```python
from build123d import *

# Parameters (mm, degrees)
F0_W     = 303
F0_H     = 174
F0_R     = 9
F0_R_2   = 7.8
F0_W_2   = 43
F0_H_2   = 80
F0_W_3   = 16.5
F0_H_3   = 7.6
F1_DEPTH = 1


with BuildPart() as f1:
    # F0 (on Top) → F1 (new body)
    with BuildSketch(Plane.XY):
        Rectangle(F0_W, F0_H)
        with Locations((121.5, -57)):
            Circle(F0_R, mode=Mode.SUBTRACT)
        with Locations((21.5, -30)):
            Circle(F0_R_2, mode=Mode.SUBTRACT)
        with Locations((51.5, -30)):
            Circle(F0_R_2, mode=Mode.SUBTRACT)
        with Locations((-110, 27)):
            Rectangle(F0_W_2, F0_H_2, mode=Mode.SUBTRACT)
        with Locations((-37, 27)):
            Rectangle(F0_W_2, F0_H_2, mode=Mode.SUBTRACT)
        with Locations((21.5, 0)):
            Circle(F0_R_2, mode=Mode.SUBTRACT)
        with Locations((51.5, 0)):
            Circle(F0_R_2, mode=Mode.SUBTRACT)
        with Locations((21.5, 30)):
            Circle(F0_R_2, mode=Mode.SUBTRACT)
        with Locations((51.5, 30)):
            Circle(F0_R_2, mode=Mode.SUBTRACT)
        with Locations((89.75, 0)):
            Rectangle(F0_W_3, F0_H_3, mode=Mode.SUBTRACT)
        with Locations((89.75, 20)):
            Rectangle(F0_W_3, F0_H_3, mode=Mode.SUBTRACT)
        with Locations((89.75, 40)):
            Rectangle(F0_W_3, F0_H_3, mode=Mode.SUBTRACT)
        with Locations((21.5, 60)):
            Circle(F0_R_2, mode=Mode.SUBTRACT)
        with Locations((51.5, 60)):
            Circle(F0_R_2, mode=Mode.SUBTRACT)
        with Locations((89.75, 60)):
            Rectangle(F0_W_3, F0_H_3, mode=Mode.SUBTRACT)
    extrude(amount=F1_DEPTH)


solid = f1.part
```
Geometry check sheet. Reference: the model listing, model coordinates, mm. Give positions to 0.01 mm unless a question says otherwise; leave off trailing zeros. Loops run counter-clockwise (first coordinate to the right, second up) from the corner with the lowest first, then second, coordinate; pieces in that order, holes last. Notation, with made-up numbers: M 36.25,-15 L 71.25,-15 A20 ccw 71.25,-5 Z; hole C 4.25,-11 d1. An arc over 180 degrees is marked long. Answer as CSV lines item,"result".
Item 1: Cross-section at B-B on y = -30. Record the cut outline in (x, z), and give its area (3 significant figures).
Values:
outline,"M -151.5,0 L 13.7,0 L 13.7,1 L -151.5,1 Z; M 29.3,0 L 43.7,0 L 43.7,1 L 29.3,1 Z; M 59.3,0 L 151.5,0 L 151.5,1 L 59.3,1 Z"
area,"272 mm²"
Item 2: Cross-section at C-C on y = -57. Record the cut outline in (x, z).
Values:
outline,"M -151.5,0 L 112.5,0 L 112.5,1 L -151.5,1 Z; M 130.5,0 L 151.5,0 L 151.5,1 L 130.5,1 Z"
Item 3: Depth check by flat-ended pin: P1, Ø12.5, axis at x = 51.5, y = 60, coming from the -Z side. Enter the tip coordinate at first touch or a pass-through.
Values:
P1,"passes through"
Item 4: Release check for a two-part mould opening along X. For faces 1 (the flat face through (-2, 1, 0)), 2 (the cylindrical face through (45.75, -24.73, 0.49)) record: pulls with the +X half, pulls with the -X half, needs draft (parallel to the pull), parting line crosses it, or undercut.
Values:
face 1,"needs draft"
face 2,"undercut"
Item 5: Material ranges on line 1 (Y direction, x = 21.5, z = 0.7); line 2 (X direction, y = 44.5, z = 0.95); line 3 (Y direction, x = 86.5, z = 0.6), recorded low to high.
Values:
line 1,"y = -87 to -37.8, -22.2 to -7.8, 7.8 to 22.2, 37.8 to 52.2, 67.8 to 87"
line 2,"x = -151.5 to -131.5, -88.5 to -58.5, -15.5 to 151.5"
line 3,"y = -87 to -3.8, 3.8 to 16.2, 23.8 to 36.2, 43.8 to 56.2, 63.8 to 87"
Item 6: Cross-section at D-D on x = 21.5. Record the cut outline in (y, z).
Values:
outline,"M -87,0 L -37.8,0 L -37.8,1 L -87,1 Z; M -22.2,0 L -7.8,0 L -7.8,1 L -22.2,1 Z; M 7.8,0 L 22.2,0 L 22.2,1 L 7.8,1 Z; M 37.8,0 L 52.2,0 L 52.2,1 L 37.8,1 Z; M 67.8,0 L 87,0 L 87,1 L 67.8,1 Z"
Item 7: Cross-section at A-A on x = -20. Record the cut outline in (y, z).
Values:
outline,"M -87,0 L -13,0 L -13,1 L -87,1 Z; M 67,0 L 87,0 L 87,1 L 67,1 Z"
